from build123d import *

# Parameters (mm, degrees)
TAP_DRILL_FOR_M5_TAP1_D = 4.2
CIRPATTERN1_COUNT       = 4
CHAMFER1_SIZE           = 0.5
CHAMFER2_SIZE           = 0.5


with BuildPart() as part:
    # Sketch1 → Revolve1 (revolve)
    with BuildSketch(Plane.XY, mode=Mode.PRIVATE) as revolve1_sk:
        Polygon((-31, 0), (-17.5, 0), (-17.5, 19), (-20, 19), (-20, 4), (-31, 4), align=None)
    revolve(revolve1_sk.sketch.rotate(Axis((0, 0, 0), (0, 1, 0)), 270), axis=Axis((0, 0, 0), (0, 1, 0)))

    # Tap Drill for M5 Tap1 (through all)
    with Locations(Plane(origin=(0, 4, 0), x_dir=(1, 0, 0), z_dir=(0, 1, 0))):
        with Locations((0, 26)):
            tap_drill_for_m5_tap1 = Hole(TAP_DRILL_FOR_M5_TAP1_D / 2)

    # CirPattern1: Tap Drill for M5 Tap1 ×4 about axis
    cirpattern1_axis = Axis((0, 0, 0), (0, 1, 0))
    for i in range(1, CIRPATTERN1_COUNT):
        add(tap_drill_for_m5_tap1.rotate(cirpattern1_axis, i * 360 / CIRPATTERN1_COUNT), mode=Mode.SUBTRACT)

    # Chamfer1
    chamfer1_edges = [part.edges().sort_by_distance(p)[0] for p in [
        (0, 19, 20),
        (0, 19, 17.5),
    ]]
    chamfer(chamfer1_edges, length=CHAMFER1_SIZE)

    # Chamfer2
    chamfer2_edges = [part.edges().sort_by_distance(p)[0] for p in [
        (0, 4, 31),
    ]]
    chamfer(chamfer2_edges, length=CHAMFER2_SIZE)


solid = part.part
Work out the finished part from the listing and answer in its coordinate system (mm). A direction names the side the tool comes from. Give positions to 0.01 mm unless a question says otherwise; leave off trailing zeros. Order: outer loops, then holes, each group sorted by start corner. A loop starts at its lowest first (then second) coordinate and runs counter-clockwise, first axis right, second up. Notation, with made-up numbers: (7, 16) -> (62, 16) arc R23 cw to (62, 53) -> close; hole circle Ø8 at (-39.75, -35.5). An arc over 180 degrees is marked (long way). Answer as a JSON object with one key per item and string values. Group by question number.
1. Section C-C on y = 6.25 is taken. Determine the outline of the cut face in (x, z).
2. A tool of negligible diameter and unlimited length cuts with its end or side. For faces 1 (the flat face through (6, 4, 20)), 2 (the cylindrical face through (-27.77, 1.97, 1.13)), from which of +Z, -Z, +X, -X, +Y, -Y can it reach the whole face along a straight path? Write none if from no direction.
3. Consider line 1 along X through (y, z) = (0.85, 0); line 2 along Y through (x, z) = (-20.5, -15); line 3 along Z through (x, y) = (-7.5, 17.5). Determine where each line is inside the solid, lowest interval first. Write a range as [from, to].
4. Section B-B on z = 0 is taken. Determine the outline of the cut face in (x, y).
5. Section A-A on x = 0 is taken. Determine the outline of the cut face in (y, z), plus the area to 3 significant figures.
6. Flat-ended cylindrical pins translate along their axes: pin 1 Ø1.5 at (x, y) = (18, 4.5) entering from +Z; pin 2 Ø1 at (x, y) = (2.5, 16) entering from +Z; pin 3 Ø6 at (x, y) = (22.5, 6.5) entering from +Z; pin 4 Ø2.5 at (x, z) = (-26, 0) entering from +Y. Find the tip coordinate at first contact, or state that the pin passes through.
7. The mould has two halves that part along X. Classify faces 3 (the cylindrical face through (-30.736, 1.726, 4.036)), 4 (the cylindrical face through (1.13, 1.97, 27.77)), 5 (the flat face through (13, 0, -13)): released by +X, released by -X, zero draft, split by the parting line, or undercut.
Result sheet:
{
 "1": {"outline": "circle Ø40 at (0, 0); hole circle Ø35 at (0, 0)"},
 "2": {"face 1": "+Y", "face 2": "+Y, -Y"},
 "3": {"line 1": "x = [-31, -28.1], [-23.9, -17.5], [17.5, 23.9], [28.1, 31]", "line 2": "y = [0, 4]", "line 3": "z = [-18.54, -15.81], [15.81, 18.54]"},
 "4": {"outline": "(-31, 0) -> (-28.1, 0) -> (-28.1, 4) -> (-30.5, 4) -> (-31, 3.5) -> close; (-23.9, 0) -> (-17.5, 0) -> (-17.5, 18.5) -> (-18, 19) -> (-19.5, 19) -> (-20, 18.5) -> (-20, 4) -> (-23.9, 4) -> close; (17.5, 0) -> (23.9, 0) -> (23.9, 4) -> (20, 4) -> (20, 18.5) -> (19.5, 19) -> (18, 19) -> (17.5, 18.5) -> close; (28.1, 0) -> (31, 0) -> (31, 3.5) -> (30.5, 4) -> (28.1, 4) -> close"},
 "5": {"outline": "(0, -31) -> (3.5, -31) -> (4, -30.5) -> (4, -28.1) -> (0, -28.1) -> close; (0, -23.9) -> (4, -23.9) -> (4, -20) -> (18.5, -20) -> (19, -19.5) -> (19, -18) -> (18.5, -17.5) -> (0, -17.5) -> close; (0, 17.5) -> (18.5, 17.5) -> (19, 18) -> (19, 19.5) -> (18.5, 20) -> (4, 20) -> (4, 23.9) -> (0, 23.9) -> close; (0, 28.1) -> (4, 28.1) -> (4, 30.5) -> (3.5, 31) -> (0, 31) -> close", "area": "149 mm^2"},
 "6": {"pin 1": "stops at z = 25.07", "pin 2": "stops at z = 19.9", "pin 3": "stops at z = 22.27", "pin 4": "passes through"},
 "7": {"face 3": "split by the parting line", "face 4": "undercut", "face 5": "zero draft"}
}
